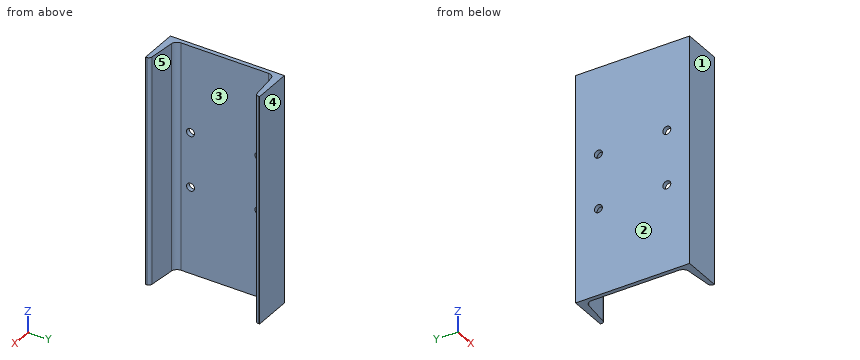
Autodesk Inventor part; units mm, degrees
ref_plane "Start Plane" through (0, 0, 0) normal (0, 0, 1) x (1, 0, 0)
ref_plane "End Plane" through (0, 0, 500) normal (0, 0, 1) x (1, 0, 0)
ref_plane "YZ Plane" through (0, 0, 0) normal (1, 0, 0) x (0, 1, 0)
ref_plane "Start Plane" through (0, 0, 0) normal (0, 0, 1) x (1, 0, 0)
ref_plane "End Plane" through (0, 0, 500) normal (0, 0, 1) x (1, 0, 0)
sketch "Sketch" plane through (0, 0, 0) normal (0, 0, 1) x (1, 0, 0)
  line L0 (-2.2, 0) -> (-2.2, 125)
  line L1 (-2.2, 125) -> (82.8, 125)
  line L2 (82.8, 125) -> (82.8, 122.2863)
  line L3 (76.5317, 115.3246) -> (19.0889, 109.2871)
  line L4 (7, 95.8611) -> (7, 0)
  line L5 (7, 0) -> (-2.2, 0) construction
  line L6 (44.9, 125) -> (44.9, 112) construction
  line L7 (82.8, 115.9834) -> (82.8, 112) construction
  line L8 (82.8, 112) -> (44.9, 112) construction
  line L9 (0, 15) -> (0, -27) construction
  line L10 (-5.539, 0) -> (16.0067, 0) construction
  line L11 (-2.2, 0) -> (-2.2, -125)
  line L12 (-2.2, -125) -> (82.8, -125)
  line L13 (82.8, -125) -> (82.8, -122.2863)
  line L14 (76.5317, -115.3246) -> (19.0889, -109.2871)
  line L15 (7, -95.8611) -> (7, 0)
  arc A0 (19.0889, 109.2871) -> (7, 95.8611) centre (20.5, 95.8611) ccw
  arc A1 (7, -95.8611) -> (19.0889, -109.2871) centre (20.5, -95.8611) ccw
  arc A2 (76.5317, 115.3246) -> (82.8, 122.2863) centre (75.8, 122.2863) ccw
  arc A3 (82.8, -122.2863) -> (76.5317, -115.3246) centre (75.8, -122.2863) ccw
  line L16 (0, 175) -> (0, -175) construction
  line L17 (-23.474, 0) -> (102.0712, 0) construction
  point P0 (7, 108.0166)
  point P1 (82.8, -115.9834)
  point P2 (7, -108.0166)
  point P3 (44.9, -125)
  point P4 (44.9, -112)
  dimension "d0" = 9.2
  dimension "d1" = 125
  dimension "d2" = 85
  dimension "d3" = 13
  dimension "d4" = 37.9
  dimension "d5" = 3.9834
  dimension "d23" = 13.5
  dimension "d24" = 7
  dimension "d25" = 2.2
extrude "Body" add sketch "Sketch" along normal up to surface (500 mm away) from surface at 0
sketch "Sketch3" plane through (0, 0, 0) normal (0, 0, 1) x (1, 0, 0)
  line L0 (0, 0) -> (10, 0)
ref_plane "Work Plane3" through (0, 0, 0) normal (0, -1, 0) x (1, 0, 0)
sketch "Sketch5" plane through (7, -95.8611, 500) normal (1, 0, 0) x (0, 0, -1)
  point P0 (190, 170.8611)
hole "Hole1" at (7, 75, 310) direction (-1, 0, 0) diameter 17.5 end through all
sketch "Sketch6" plane through (7, -95.8611, 500) normal (1, 0, 0) x (0, 0, -1)
  point P0 (310, 170.8611)
hole "Hole2" at (7, 75, 190) direction (-1, 0, 0) diameter 17.5 end through all
sketch "Sketch7" plane through (7, -95.8611, 500) normal (1, 0, 0) x (0, 0, -1)
  point P0 (190, 20.8611)
hole "Hole3" at (7, -75, 310) direction (-1, 0, 0) diameter 17.5 end through all
sketch "Sketch8" plane through (7, -95.8611, 500) normal (1, 0, 0) x (0, 0, -1)
  point P0 (310, 20.8611)
hole "Hole4" at (7, -75, 190) direction (-1, 0, 0) diameter 17.5 end through all
sketch "Sketch4" plane through (0, 0, 0) normal (0, -1, 0) x (1, 0, 0)
  line L0 (-2, 0) -> (12, 0)
  line L1 (-2, 500) -> (12, 500)
  dimension "d29" = 500
equation "\"d0\" = G_T"
equation "\"d1\" = 0.5 * G_H"
equation "\"d2\" = G_W"
equation "\"d3\" = G_T1"
equation "\"d4\" = G_C"
equation "\"d23\" = G_IR"
equation "\"d24\" = G_ER"
equation "\"d25\" = ex"
equation "\"d6\" = G_L"
equation "\"G_W\" = 85"
equation "\"G_H\" = 250"
equation "\"G_T\" = 9.2"
equation "\"G_T1\" = 13"
equation "\"G_NG\" = 0.105104"
equation "\"G_ER\" = 7"
equation "\"G_IR\" = 13.5"
equation "\"G_C\" = 37.9"
equation "\"G_L\" = d29"
equation "\"ex\" = 2.2"
equation "\"G_OFFSET_START\" = 0"
equation "\"G_OFFSET_END\" = 0"
properties part number "ISO 657/11 - CH 250 x 34 - 500" material "Steel, Mild"
Design review of the part built by this model. Coordinates are the model's own, in mm. Face numbers are marked on the shaded views. A direction names the side the tool comes from. Coordinates: 2 decimals unless noted, no trailing zeros. Order: outer loops, then holes, each group sorted by start corner. A loop starts at its lowest first (then second) coordinate and runs counter-clockwise, first axis right, second up.
1) Mouldability with a two-part tool opening along Y and no side actions: class the marked faces 1, 2 and 3 as +Y half, -Y half, draft (parallel to the pull), parting line (faces both ways), or undercut.
2) Take a section at A-A, the plane y = 75. Give the boundary of the cut face in (x, z).
3) Clearance check with flat-ended pins moving along their axes: pin 1 (20 mm diameter, centred on y = 75, z = 190, fed in from +X); pin 2 (16 mm diameter, centred on y = -75, z = 310, fed in from +X). State where each tip first meets the part, or that it passes through.
4) Take a section at C-C, the plane x = 24.5. Give the boundary of the cut face in (y, z), and give its area (3 significant figures).
5) Wall thickness on line 1 along Y through (x, z) = (3, 190); line 2 along Z through (x, y) = (0, 75); line 3 along X through (y, z) = (-20.5, 473): over which ranges is each line inside the solid? List them lowest first.
6) For the marked faces 4 and 5, list the 3-axis set-ups (+Z, -Z, +X, -X, +Y, -Y) from which the entire face can be reached by the end or side of a thin tool; tool diameter is ignored.
7) Take a section at D-D, the plane x = 55. Give the boundary of the cut face in (y, z), and give its area (3 significant figures).
8) Take a section at B-B, the plane z = 190. Give the boundary of the cut face in (x, y), and give its area (3 significant figures).
Returned:
1. face 1: -Y half
1. face 2: draft
1. face 3: undercut
2. outline: (-2.2, 0) - (7, 0) - (7, 181.25) - (-2.2, 181.25) - close; (-2.2, 198.75) - (7, 198.75) - (7, 301.25) - (-2.2, 301.25) - close; (-2.2, 318.75) - (7, 318.75) - (7, 500) - (-2.2, 500) - close
3. pin 1: stops at x = 7
3. pin 2: passes through
4. outline: (-125, 0) - (-109.86, 0) - (-109.86, 500) - (-125, 500) - close; (109.86, 0) - (125, 0) - (125, 500) - (109.86, 500) - close
4. area: 15,100 mm2
5. line 1: y = -125 to -83.75, -66.25 to 66.25, 83.75 to 125
5. line 2: z = 0 to 181.25, 198.75 to 301.25, 318.75 to 500
5. line 3: x = -2.2 to 7
6. face 4: +Z, -Z, +X, -X, +Y
6. face 5: +Z, -Z, +X
7. outline: (-125, 0) - (-113.06, 0) - (-113.06, 500) - (-125, 500) - close; (113.06, 0) - (125, 0) - (125, 500) - (113.06, 500) - close
7. area: 11,900 mm2
8. outline: (-2.2, -125) - (82.8, -125) - (82.8, -122.29) arc R7 ccw to (76.53, -115.32) - (19.09, -109.29) arc R13.5 cw to (7, -95.86) - (7, -83.75) - (-2.2, -83.75) - close; (-2.2, -66.25) - (7, -66.25) - (7, 66.25) - (-2.2, 66.25) - close; (-2.2, 83.75) - (7, 83.75) - (7, 95.86) arc R13.5 cw to (19.09, 109.29) - (76.53, 115.32) arc R7 ccw to (82.8, 122.29) - (82.8, 125) - (-2.2, 125) - close
8. area: 3,990 mm2
